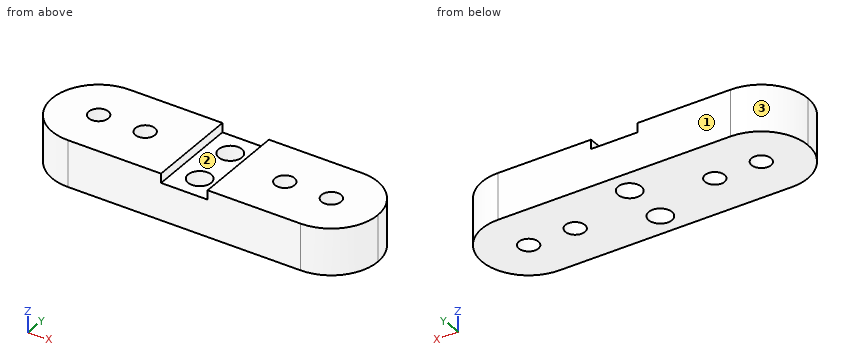
```python
from build123d import *

# Parameters (mm, degrees)
ESQUISSE1_R             = 2.5
BOSS_EXTRU_1_DEPTH      = 10
CONG_1_R                = 10
TROU_TARAUD_M5X0_81_D   = 4.2
ESQUISSE5_W             = 10
ESQUISSE5_H             = 20
ENL_V_MAT_EXTRU_1_DEPTH = 2


with BuildPart() as part:
    # Esquisse1 → Boss.-Extru.1 (new body)
    with BuildSketch(Plane.XY):
        Polygon((50, 20), (0, 20), (0, 0), (50, 0), (60, 0), (70, 0), (70, 20), (60, 20), align=None)
        with Locations((35, 5)):
            Circle(ESQUISSE1_R, mode=Mode.SUBTRACT)
        with Locations((35, 15)):
            Circle(ESQUISSE1_R, mode=Mode.SUBTRACT)
    extrude(amount=BOSS_EXTRU_1_DEPTH)

    # Congé1
    cong_1_edges = [part.edges().sort_by_distance(p)[0] for p in [
        (0, 0, 5),
        (0, 20, 5),
        (70, 0, 5),
        (70, 20, 5),
    ]]
    fillet(cong_1_edges, radius=CONG_1_R - 0.0001)  # a hair under: the kernel refuses the full size

    # Trou taraudé M5x0.81 (through all)
    with Locations(Plane.XY.offset(10)):
        with Locations((50, 10), (60, 10), (10, 10), (20, 10)):
            Hole(TROU_TARAUD_M5X0_81_D / 2)

    # Esquisse5 → Enlèv. mat.-Extru.1 (cut)
    with BuildSketch(Plane.XY.offset(10)):
        with Locations((35, 10)):
            Rectangle(ESQUISSE5_W, ESQUISSE5_H)
    extrude(amount=-ENL_V_MAT_EXTRU_1_DEPTH, mode=Mode.SUBTRACT)


solid = part.part
```
Here's how the part is built. I have some questions about the finished solid (model axes, mm). Face numbers are marked on the shaded views. Round coordinates to 2 decimals unless told otherwise and drop trailing zeros. Loops run counter-clockwise (first coordinate to the right, second up) from the corner with the lowest first, then second, coordinate; pieces in that order, holes last. Notation, with made-up numbers: (39.25, -35) -> (84.25, -35) arc R12 cw to (84.25, -20) -> close; hole circle Ø7 at (53.5, -14.75). An arc over 180 degrees is marked (long way). Answer as CSV lines item,"result". Start each with the question number.
1. If we mould it in two halves opening along X, with no side actions, what happens to the marked faces 1, 2 and 3? For each: pulls with the +X half, pulls with the -X half, needs draft (parallel to the pull), parting line crosses it, or undercut.
2. Imagine slicing it at C-C on y = 14.25. Write out the boundary of the cut face in (x, z), plus the area to 3 significant figures.
3. I'm going to push flat-ended pins straight in: P1, Ø1.6, axis at y = 12.5, z = 8.5, coming from the +X side; P2, Ø1, axis at x = 8.5, z = 8, coming from the -Y side; P3, Ø3.5, axis at x = 10, y = 10, coming from the -Z side; P4, Ø1, axis at y = 11, z = 9.5, coming from the -X side. Where does each tip first touch, or does it pass through?
4. I need wall thicknesses on probe 1 along Y at (x, z) = (10, 5.75); probe 2 along Y at (x, z) = (35, 3); probe 3 along X at (y, z) = (11, 6.5). Which ranges of each line are inside material? Lowest first, please. Write a range as from..to.
5. Imagine slicing it at A-A on x = 50. Write out the boundary of the cut face in (y, z), plus the area to 3 significant figures.
6. Imagine slicing it at D-D on x = 35. Write out the boundary of the cut face in (y, z), plus the area to 3 significant figures.
7. Imagine slicing it at B-B on z = 4. State how many separate pieces and enclosed holes the cut face has, plus the area to 3 significant figures.
Solution:
1,face 1,"needs draft"
1,face 2,"undercut"
1,face 3,"pulls with the -X half"
2,outline,"(0.95, 0) -> (32.62, 0) -> (32.62, 8) -> (30, 8) -> (30, 10) -> (0.95, 10) -> close; (37.38, 0) -> (69.05, 0) -> (69.05, 10) -> (40, 10) -> (40, 8) -> (37.38, 8) -> close"
2,area,"623 mm²"
3,P1,"x = 69.85"
3,P2,"y = 0.05"
3,P3,"through"
3,P4,"x = 0.01"
4,probe 1,"0..7.9, 12.1..20"
4,probe 2,"0..2.5, 7.5..12.5, 17.5..20"
4,probe 3,"0.05..8.15, 11.85..18.15, 21.85..48.15, 51.85..58.15, 61.85..69.95"
5,outline,"(0, 0) -> (7.9, 0) -> (7.9, 10) -> (0, 10) -> close; (12.1, 0) -> (20, 0) -> (20, 10) -> (12.1, 10) -> close"
5,area,"158 mm²"
6,outline,"(0, 0) -> (2.5, 0) -> (2.5, 8) -> (0, 8) -> close; (7.5, 0) -> (12.5, 0) -> (12.5, 8) -> (7.5, 8) -> close; (17.5, 0) -> (20, 0) -> (20, 8) -> (17.5, 8) -> close"
6,area,"80.0 mm²"
7,separate pieces,"1"
7,enclosed holes,"6"
7,area,"1,220 mm²"
